from build123d import *

# Parameters (mm, degrees)
SKETCH1_W           = 50.04
SKETCH1_H           = 30.04
SKETCH1_W_2         = 40.04
SKETCH1_H_2         = 20.04
SKETCH1_W_3         = 5
BOSS_EXTRUDE2_DEPTH = 28
SKETCH2_W           = 50.04
SKETCH2_H           = 30.04
SKETCH2_W_2         = 17.52
SKETCH2_H_2         = 20.04
BOSS_EXTRUDE3_DEPTH = 5
SKETCH3_W           = 5
SKETCH3_H           = 20.04
CUT_EXTRUDE1_DEPTH  = 27
SKETCH4_W           = 5
SKETCH4_H           = 20.04
CUT_EXTRUDE3_DEPTH  = 27
SKETCH5_W           = 40.04
SKETCH5_H           = 28.980890752
CUT_EXTRUDE4_DEPTH  = 47
SKETCH6_W           = 5
SKETCH6_H           = 5
BOSS_EXTRUDE4_DEPTH = 45
CUT_EXTRUDE5_DEPTH  = 66
SKETCH8_W           = 5
SKETCH8_H           = 3
BOSS_EXTRUDE5_DEPTH = 29
SKETCH9_W           = 40.04
SKETCH9_H           = 5
CUT_EXTRUDE6_DEPTH  = 51
SKETCH10_W          = 40.04
SKETCH10_H          = 3
BOSS_EXTRUDE6_DEPTH = 5
SKETCH12_W          = 40.04
SKETCH12_H          = 3
BOSS_EXTRUDE7_DEPTH = 5
FILLET1_R           = 2
SKETCH13_W          = 23
SKETCH13_H          = 0.02
CUT_EXTRUDE7_DEPTH  = 87
SKETCH14_W          = 5
SKETCH14_H          = 5
SKETCH14_R          = 1.5
BOSS_EXTRUDE8_DEPTH = 5
FILLET2_R           = 2


with BuildPart() as part:
    # Sketch1 → Boss-Extrude2 (new body)
    with BuildSketch(Plane.XY):
        with Locations((20.02, -10.02)):
            Rectangle(SKETCH1_W, SKETCH1_H)
        with Locations((20.02, -10.02)):
            Rectangle(SKETCH1_W_2, SKETCH1_H_2, mode=Mode.SUBTRACT)
        with Locations((20.02, -10.02)):
            Rectangle(SKETCH1_W_3, SKETCH1_H_2)
    extrude(amount=BOSS_EXTRUDE2_DEPTH)

    # Sketch2 → Boss-Extrude3 (add)
    with BuildSketch(Plane(origin=(0, 0, 0), x_dir=(-1, 0, 0), z_dir=(0, 0, -1))):
        with Locations((-20.02, -10.02)):
            Rectangle(SKETCH2_W, SKETCH2_H)
        with Locations((-31.28, -10.02)):
            Rectangle(SKETCH2_W_2, SKETCH2_H_2, mode=Mode.SUBTRACT)
        with Locations((-8.76, -10.02)):
            Rectangle(SKETCH2_W_2, SKETCH2_H_2, mode=Mode.SUBTRACT)
    extrude(amount=BOSS_EXTRUDE3_DEPTH)

    # Sketch3 → Cut-Extrude1 (cut)
    with BuildSketch(Plane.XY.offset(28)):
        with Locations((20.02, -10.02)):
            Rectangle(SKETCH3_W, SKETCH3_H)
    extrude(amount=-CUT_EXTRUDE1_DEPTH, mode=Mode.SUBTRACT)

    # Sketch4 → Cut-Extrude3 (cut)
    with BuildSketch(Plane(origin=(0, 0, -5), x_dir=(-1, 0, 0), z_dir=(0, 0, -1))):
        with Locations((-42.54, -10.02)):
            Rectangle(SKETCH4_W, SKETCH4_H)
        with Locations((2.5, -10.02)):
            Rectangle(SKETCH4_W, SKETCH4_H)
    extrude(amount=-CUT_EXTRUDE3_DEPTH, mode=Mode.SUBTRACT)

    # Sketch5 → Cut-Extrude4 (cut)
    with BuildSketch(Plane(origin=(0, 5, 0), x_dir=(1, 0, 0), z_dir=(0, 1, 0))):
        with Locations((20.02, -13.509554624)):
            Rectangle(SKETCH5_W, SKETCH5_H)
    extrude(amount=-CUT_EXTRUDE4_DEPTH, mode=Mode.SUBTRACT)

    # Sketch6 → Boss-Extrude4 (add)
    with BuildSketch(Plane(origin=(0, 0, 0), x_dir=(0, 0, -1), z_dir=(1, 0, 0))):
        with Locations((-11.5, 2.5)):
            Rectangle(SKETCH6_W, SKETCH6_H)
        with Locations((-11.5, -22.54)):
            Rectangle(SKETCH6_W, SKETCH6_H)
    extrude(amount=BOSS_EXTRUDE4_DEPTH)

    # Sketch7 → Cut-Extrude5 (cut)
    with BuildSketch(Plane(origin=(45.04, 0, 0), x_dir=(0, 0, -1), z_dir=(1, 0, 0))):
        Polygon((-28, -25.04), (-18, -25.04), (-18, -20.04), (-22, -20.04), (-22, 0), (-18, 0), (-18, 5), (-28, 5), align=None)
    extrude(amount=-CUT_EXTRUDE5_DEPTH, mode=Mode.SUBTRACT)

    # Sketch8 → Boss-Extrude5 (add)
    with BuildSketch(Plane.XZ.offset(25.04)):
        with Locations((-2.5, 8.509554624)):
            Rectangle(SKETCH8_W, SKETCH8_H)
        with Locations((42.54, 8.509554624)):
            Rectangle(SKETCH8_W, SKETCH8_H)
    extrude(amount=-BOSS_EXTRUDE5_DEPTH)

    # Sketch9 → Cut-Extrude6 (cut)
    with BuildSketch(Plane(origin=(0, -25.04, 0), x_dir=(-1, 0, 0), z_dir=(0, -1, 0))):
        with Locations((-20.02, -11.5)):
            Rectangle(SKETCH9_W, SKETCH9_H)
    extrude(amount=-CUT_EXTRUDE6_DEPTH, mode=Mode.SUBTRACT)

    # Sketch10 → Boss-Extrude6 (add)
    with BuildSketch(Plane.XZ.offset(25.04)):
        with Locations((20.02, 8.509554624)):
            Rectangle(SKETCH10_W, SKETCH10_H)
    extrude(amount=-BOSS_EXTRUDE6_DEPTH)

    # Sketch12 → Boss-Extrude7 (add)
    with BuildSketch(Plane(origin=(0, 5, 0), x_dir=(1, 0, 0), z_dir=(0, 1, 0))):
        with Locations((20.02, -8.509554624)):
            Rectangle(SKETCH12_W, SKETCH12_H)
    extrude(amount=-BOSS_EXTRUDE7_DEPTH)

    # Fillet1
    fillet1_edges = [part.edges().sort_by_distance(p)[0] for p in [
        (40.04, 2.5, 18),
        (0, 2.5, 18),
        (-5, 2.5, 18),
        (40.04, -22.54, 18),
        (0, -22.54, 18),
        (-5, -22.54, 18),
        (45.04, -22.54, 18),
        (45.04, 2.5, 18),
        (45.04, 2.5, -5),
        (-5, -22.54, -5),
        (45.04, -22.54, -5),
        (-5, 2.5, -5),
    ]]
    fillet(fillet1_edges, radius=FILLET1_R)

    # Sketch13 → Cut-Extrude7 (cut)
    with BuildSketch(Plane(origin=(45.04, 0, 0), x_dir=(0, 0, -1), z_dir=(1, 0, 0))):
        with Locations((-6.5, -25.03)):
            Rectangle(SKETCH13_W, SKETCH13_H)
        with Locations((-6.5, 4.99)):
            Rectangle(SKETCH13_W, SKETCH13_H)
    extrude(amount=-CUT_EXTRUDE7_DEPTH, mode=Mode.SUBTRACT)

    # Sketch14 → Boss-Extrude8 (add)
    with BuildSketch(Plane(origin=(45.04, 0, 0), x_dir=(0, 0, -1), z_dir=(1, 0, 0))):
        with Locations((-6.5, -27.52)):
            Rectangle(SKETCH14_W, SKETCH14_H)
        with Locations((-6.5, -27.52)):
            Circle(SKETCH14_R, mode=Mode.SUBTRACT)
        with Locations((-6.5, 7.48)):
            Rectangle(SKETCH14_W, SKETCH14_H)
        with Locations((-6.5, 7.48)):
            Circle(SKETCH14_R, mode=Mode.SUBTRACT)
    extrude(amount=-BOSS_EXTRUDE8_DEPTH)

    # Fillet2
    fillet2_edges = [part.edges().sort_by_distance(p)[0] for p in [
        (42.54, -30.02, 4),
        (42.54, -30.02, 9),
        (42.54, 9.98, 4),
        (42.54, 9.98, 9),
    ]]
    fillet(fillet2_edges, radius=FILLET2_R)


solid = part.part
Design review of the part built by this model. Coordinates are the model's own, in mm. A direction names the side the tool comes from. Coordinates: 2 decimals unless noted, no trailing zeros. Order: outer loops, then holes, each group sorted by start corner. A loop starts at its lowest first (then second) coordinate and runs counter-clockwise, first axis right, second up.
Item 1: Take a section at C-C, the plane x = 2. Write out the cut boundary in (y, z), then the cut area to 3 significant figures.
Item 2: Take a section at B-B, the plane z = 14.25. Write out the cut boundary in (x, y), then the cut area to 3 significant figures.
Item 3: For faces 1 (the flat face through (-3, -10, 10.01)), 2 (the cylindrical face through (-0.6, -22.5, 17.43)), 3 (the flat face through (40.04, 4, 4)), list the 3-axis set-ups (+Z, -Z, +X, -X, +Y, -Y) from which the entire face can be reached by the end or side of a thin tool; tool diameter is ignored.
Item 4: The part is to be moulded in two halves that separate along X. For faces 4 (the flat face through (40.04, 3, 13)), 5 (the flat face through (45.04, -10, 8)), 6 (the flat face through (43, -10, 7.01)), say which applies: pulls with the +X half, pulls with the -X half, needs draft (parallel to the pull), parting line crosses it, or undercut.
Item 5: Take a section at A-A, the plane y = -16. Write out the cut boundary in (x, z).
Item 6: For line 1 (Y direction, x = 44.05, z = 6.5); line 2 (Y direction, x = 11, z = 8); line 3 (X direction, y = 2, z = 14), list the stretches that pass through material, from the lowest coordinate up.
Item 7: For pin 1 Ø1 at (x, z) = (34.5, -2.5) entering from +Y; pin 2 Ø4.5 at (y, z) = (-7.5, -3) entering from +X; pin 3 Ø7 at (x, z) = (13, 7.5) entering from -Y; pin 4 Ø5 at (y, z) = (-7, 13.5) entering from +X, all flat-tipped, find the tip position at first contact; note any pin that passes through.
Item 8: Take a section at D-D, the plane y = -23.5. Write out the cut boundary in (x, z).
The answers:
1. outline: (-25.02, -5) - (-20.04, -5) - (-20.04, -0.98) - (-25.02, -0.98) - close; (-25.02, 7.01) - (-20.04, 7.01) - (-20.04, 10.01) - (-25.02, 10.01) - close; (0, -5) - (4.98, -5) - (4.98, -0.98) - (0, -0.98) - close; (0, 7.01) - (4.98, 7.01) - (4.98, 10.01) - (0, 10.01) - close
1. area: 69.9 mm2
2. outline: (-5, -25.02) - (0, -25.02) - (0, -20.04) - (-5, -20.04) - close; (-5, 0) - (0, 0) - (0, 4.98) - (-5, 4.98) - close; (40.04, -25.02) - (45.04, -25.02) - (45.04, -20.04) - (40.04, -20.04) - close; (40.04, 0) - (45.04, 0) - (45.04, 4.98) - (40.04, 4.98) - close
2. area: 99.6 mm2
3. face 1: +Z, +X, -X
3. face 2: +Z, +Y, -Y
3. face 3: +Y
4. face 4: undercut
4. face 5: pulls with the +X half
4. face 6: needs draft
5. outline: (-5, 7.01) - (0, 7.01) - (0, 10.01) - (-5, 10.01) - close; (17.52, -5) - (22.52, -5) - (22.52, -0.98) - (17.52, -0.98) - close; (40.04, 7.01) - (45.04, 7.01) - (45.04, 10.01) - (40.04, 10.01) - close
6. line 1: y = -30.02 to -29.02, -26.02 to -20.04, 0 to 5.98, 8.98 to 9.98
6. line 2: y = -25.02 to -20.04, 0 to 4.98
6. line 3: x = -5 to 0, 40.04 to 45.04
7. pin 1: stops at y = 4.98
7. pin 2: stops at x = 22.52
7. pin 3: stops at y = -25.02
7. pin 4: passes through
8. outline: (-5, -3) arc R2 ccw to (-3, -5) - (43.04, -5) arc R2 ccw to (45.04, -3) - (45.04, 16) arc R2 ccw to (43.04, 18) - (42.04, 18) arc R2 ccw to (40.04, 16) - (40.04, 10.01) - (0, 10.01) - (0, 16) arc R2 ccw to (-2, 18) - (-3, 18) arc R2 ccw to (-5, 16) - close; hole (0, -0.98) - (40.04, -0.98) - (40.04, 7.01) - (0, 7.01) - close
